Read the model definition and answer for the solid it produces. Units are mm, in the model's axes. Give positions to 0.01 mm unless a question says otherwise; leave off trailing zeros. Order: outer loops, then holes, each group sorted by start corner. A loop starts at its lowest first (then second) coordinate and runs counter-clockwise, first axis right, second up. Notation, with made-up numbers: (67, -17) -> (99, -17) arc R21 ccw to (99, 11) -> close; hole circle Ø11 at (-0.75, -36). An arc over 180 degrees is marked (long way). Use one line per item in the form item = value.
```python
from build123d import *

# Parameters (mm, degrees)
BOSS_EXTRUDE1_DEPTH                                = 3.4925
CUT_EXTRUDE1_DEPTH                                 = 3.96875
CSK_FOR_10_FLAT_HEAD_SOCKET_CAP_SCREW1_D           = 5.1054
CSK_FOR_10_FLAT_HEAD_SOCKET_CAP_SCREW1_CSINK_D     = 10.4394
CSK_FOR_10_FLAT_HEAD_SOCKET_CAP_SCREW1_CSINK_ANGLE = 82
CUT_EXTRUDE2_DEPTH                                 = 245.141012004
CUT_EXTRUDE2_DEPTH_BACK                            = 245.141012004
SKETCH3_3_R                                        = 2.38125
F_8_32_TAPPED_HOLE2_D                              = 3.4544


with BuildPart() as part:
    # Sketch2 → Boss-Extrude1 (new, symmetric)
    with BuildSketch(Plane(origin=(0, 0, 0), x_dir=(0, 0, -1), z_dir=(1, 0, 0))):
        with BuildLine():
            ThreePointArc((153.979316793, 88.9), (177.123417321, -15.496291061), (136.202701987, -114.287637002))
            ThreePointArc((136.202701987, -114.287637002), (137.768063771, -132.179804073), (155.660230842, -130.614442288))
            ThreePointArc((155.660230842, -130.614442288), (202.426762652, -17.710046926), (175.976362049, 101.6))
            ThreePointArc((175.976362049, 101.6), (158.627839421, 106.248522628), (153.979316793, 88.9))
        make_face()
    extrude(amount=BOSS_EXTRUDE1_DEPTH, both=True)

    # Sketch3 → Cut-Extrude1 (cut, symmetric)
    with BuildSketch(Plane.ZY.offset(-3.4925)):
        with BuildLine():
            ThreePointArc((-161.5408011, 93.265625), (-186.249876712, -10.241613709), (-150.340665851, -110.415539748))
            ThreePointArc((-150.340665851, -110.415539748), (-147.011863227, -110.925222209), (-146.502180766, -107.596419585))
            ThreePointArc((-146.502180766, -107.596419585), (-181.494560711, -9.980125699), (-157.416355114, 90.884375))
            ThreePointArc((-157.416355114, 90.884375), (-158.287953107, 94.137222993), (-161.5408011, 93.265625))
        make_face()
    extrude(amount=CUT_EXTRUDE1_DEPTH, both=True, mode=Mode.SUBTRACT)

    # CSK for #10 Flat Head Socket Cap Screw1 (through all)
    with Locations(Plane(origin=(3.4925, 0, 0), x_dir=(0, 0, -1), z_dir=(1, 0, 0))):
        with Locations((175.529160654, 81.850591843), (192.938008153, 16.879888477), (187.075684407, -50.12677856), (158.649272178, -111.08741631)):
            CounterSinkHole(CSK_FOR_10_FLAT_HEAD_SOCKET_CAP_SCREW1_D / 2, CSK_FOR_10_FLAT_HEAD_SOCKET_CAP_SCREW1_CSINK_D / 2, counter_sink_angle=CSK_FOR_10_FLAT_HEAD_SOCKET_CAP_SCREW1_CSINK_ANGLE)

    # Sketch3<3> → Cut-Extrude2 (cut, two sides: drawn at the far end of the back side and taken through both)
    with BuildSketch(Plane.ZY.offset(-3.4925).offset(-CUT_EXTRUDE2_DEPTH_BACK)):
        with Locations((-141.0670842, -118.369338324)):
            Circle(SKETCH3_3_R)
    extrude(amount=CUT_EXTRUDE2_DEPTH + CUT_EXTRUDE2_DEPTH_BACK, mode=Mode.SUBTRACT)

    # #8-32 Tapped Hole2 (through all)
    with Locations(Plane(origin=(3.4925, 0, 0), x_dir=(0, 0, -1), z_dir=(1, 0, 0))):
        with Locations((167.727470078, 96.8375), (189.67379492, 39.164488321), (175.529160654, -81.850591843), (192.365438936, -22.484295143)):
            Hole(F_8_32_TAPPED_HOLE2_D / 2)


solid = part.part
```
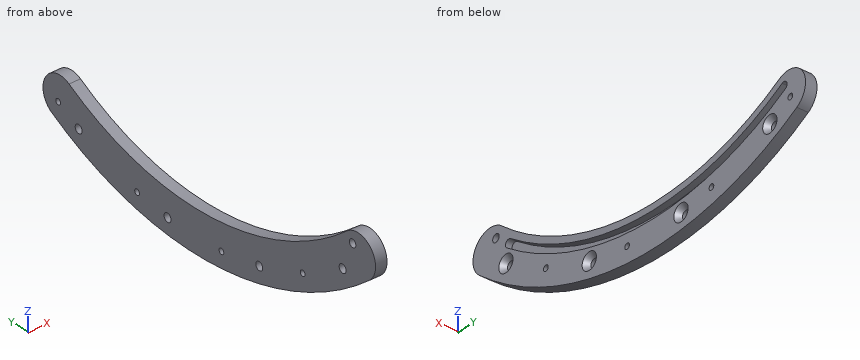
Item 1: The part is cut by section A-A on x = -1.75. State how many separate pieces and enclosed holes the cut face has, and give its area (3 significant figures).
Checks:
separate_pieces = 1
enclosed_holes = 9
area = 6,280 mm²
Item 2: The part is cut by section B-B on y = -6. Give the vertices of the cut face in (x, z), and give its area (3 significant figures).
Checks:
outline = (-3.49, -203.11) -> (3.49, -203.11) -> (3.49, -186.43) -> (-0.48, -186.43) -> (-0.48, -181.67) -> (3.49, -181.67) -> (3.49, -177.7) -> (-3.49, -177.7) -> close
area = 159 mm²
Item 3: Straight lines are drawn through the part: L1, parallel to Z at x = 2.5, y = -47; L2, parallel to X at y = -63, z = -175.5; L3, parallel to Z at x = -0.25, y = -39.5 (3 decimals). For each, find the intervals that lie inside material, in ascending order. Write a range as from..to.
Checks:
L1 = -197.69..-190.11, -184.04..-180.51, -175.59..-171.48
L2 = -3.49..-0.48
L3 = -199.324..-182.301, -177.425..-173.357
Item 4: Given pin 1 Ø6 at (y, z) = (16.88, -192.94) entering from +X; pin 2 Ø2 at (x, y) = (-2.5, -68) entering from -Z; pin 3 Ø2 at (x, y) = (0, 78.5) entering from +Z, each flat-ended and moving along its own axis, determine where each tip first touches the part or whether it passes through.
Checks:
pin_1 = 0.94
pin_2 = -191.84
pin_3 = -159.04
